CAD build for the part. Positions are in the model's coordinates, mm. Face numbers are marked on the shaded views. A direction names the side the tool comes from. Round coordinates to 2 decimals unless told otherwise and drop trailing zeros. Loops run counter-clockwise (first coordinate to the right, second up) from the corner with the lowest first, then second, coordinate; pieces in that order, holes last.
from build123d import *

# Parameters (mm, degrees)
SKETCH1_R           = 1.75
BOSS_EXTRUDE1_DEPTH = 11.738
CUT_EXTRUDE1_DEPTH  = 2.3
SKETCH3_R           = 2.54
BOSS_EXTRUDE2_DEPTH = 4.738


with BuildPart() as part:
    # Sketch1 → Boss-Extrude1 (new body)
    with BuildSketch(Plane(origin=(0, 0, 0), x_dir=(1, 0, 0), z_dir=(0, 1, 0))):
        Circle(SKETCH1_R)
    extrude(amount=BOSS_EXTRUDE1_DEPTH)

    # Sketch2 → Cut-Extrude1 (cut)
    with BuildSketch(Plane(origin=(0, 11.738, 0), x_dir=(1, 0, 0), z_dir=(0, 1, 0))):
        with BuildLine():
            Line((-1, -1.436140662), (-1, 1.436140662))
            ThreePointArc((-1, 1.436140662), (-1.75, 0), (-1, -1.436140662))
        make_face()
        with BuildLine():
            ThreePointArc((1.75, 0), (1.551209206, 0.810092587), (1, 1.436140662))
            Line((1, 1.436140662), (1, -1.436140662))
            ThreePointArc((1, -1.436140662), (1.551209206, -0.810092587), (1.75, 0))
        make_face()
    extrude(amount=-CUT_EXTRUDE1_DEPTH, mode=Mode.SUBTRACT)

    # Sketch3 → Boss-Extrude2 (add)
    with BuildSketch(Plane.XZ):
        Circle(SKETCH3_R)
    extrude(amount=-BOSS_EXTRUDE2_DEPTH)


solid = part.part
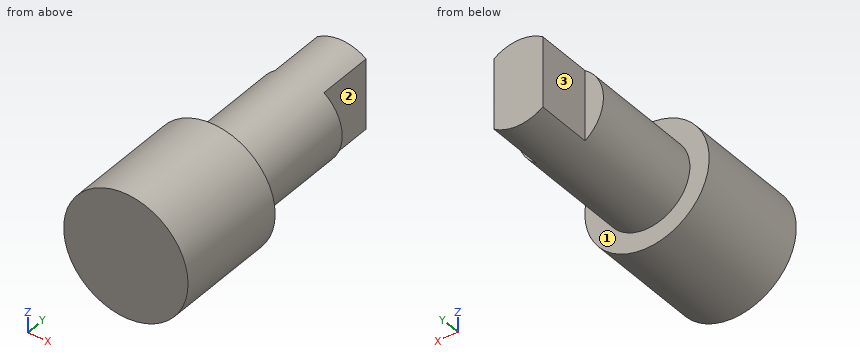
Item 1: Flat gauge pins, fed straight in: P1, Ø1, axis at y = 4, z = 1, coming from the -X side; P2, Ø2.5, axis at y = 10, z = -0.5, coming from the +X side; P3, Ø0.8, axis at x = 1.5, z = 0, coming from the +Y side. Where does each tip first touch, or does it go through?
Verdict:
P1: stops at x = -2.49
P2: stops at x = 1.75
P3: stops at y = 9.44
Item 2: Wall check: L1, parallel to Y at x = -1.25, z = -0.5; L2, parallel to Y at x = -2.15, z = 0.25; L3, parallel to X at y = 3.5, z = -0.1. Give the ranges that are in metal, low to high.
Verdict:
L1: y = 0 to 9.44
L2: y = 0 to 4.74
L3: x = -2.54 to 2.54
Item 3: Cut at C-C (y = 8). List the corners of the cut face in (x, z).
Verdict:
outline: circle Ø3.5 at (0, 0)
Item 4: Cut at A-A (x = 0). List the corners of the cut face in (y, z), plus the area to 3 significant figures.
Verdict:
outline: (0, -2.54) - (4.74, -2.54) - (4.74, -1.75) - (11.74, -1.75) - (11.74, 1.75) - (4.74, 1.75) - (4.74, 2.54) - (0, 2.54) - close
area: 48.6 mm2
Item 5: Cut at D-D (x = -1.55). List the corners of the cut face in (y, z).
Verdict:
outline: (0, -2.01) - (4.74, -2.01) - (4.74, -0.81) - (9.44, -0.81) - (9.44, 0.81) - (4.74, 0.81) - (4.74, 2.01) - (0, 2.01) - close
Item 6: 3-axis set-ups, long thin cutter, end or side, ignore diameter. For the marked faces 1, 2 and 3: which of +Z, -Z, +X, -X, +Y, -Y reach the whole face in a straight line?
Verdict:
face 1: +Y
face 2: +Z, -Z, +X, +Y
face 3: +Z, -Z, -X, +Y
Item 7: Cut at B-B (z = 0). List the corners of the cut face in (x, y), plus the area to 3 significant figures.
Verdict:
outline: (-2.54, 0) - (2.54, 0) - (2.54, 4.74) - (1.75, 4.74) - (1.75, 9.44) - (1, 9.44) - (1, 11.74) - (-1, 11.74) - (-1, 9.44) - (-1.75, 9.44) - (-1.75, 4.74) - (-2.54, 4.74) - close
area: 45.1 mm2
